from build123d import *

# Parameters (mm, degrees)
ESBO_O1_R                = 2
RESSALTO_EXTRUS_O1_DEPTH = 3.5
ESBO_O2_R                = 1
CORTE_EXTRUS_O1_DEPTH    = 6.573642863


with BuildPart() as part:
    # Esboço1 → Ressalto-extrusão1 (new body)
    with BuildSketch(Plane.XY):
        Circle(ESBO_O1_R)
        with BuildLine():
            ThreePointArc((-1.509485071, 1.312042233), (-1.175570505, 1.618033989), (-0.781369776, 1.84104896))
            Line((-0.781369776, 1.84104896), (-0.871690079, 1.965364192))
            ThreePointArc((-0.871690079, 1.965364192), (-1.253664041, 2.349535361), (-1.734231738, 2.599627912))
            ThreePointArc((-1.734231738, 2.599627912), (-1.836828913, 2.528178107), (-1.936485986, 2.452681599))
            ThreePointArc((-1.936485986, 2.452681599), (-1.847137421, 1.918351711), (-1.599805374, 1.436357465))
            Line((-1.599805374, 1.436357465), (-1.509485071, 1.312042233))
        make_face()
        with BuildLine():
            ThreePointArc((-0.45, 1.948717527), (0, 2), (0.45, 1.948717527))
            Line((0.45, 1.948717527), (0.45, 2.102379604))
            ThreePointArc((0.45, 2.102379604), (0.36678672, 2.63769927), (0.125, 3.122498999))
            ThreePointArc((0.125, 3.122498999), (0, 3.125), (-0.125, 3.122498999))
            ThreePointArc((-0.125, 3.122498999), (-0.36678672, 2.63769927), (-0.45, 2.102379604))
            Line((-0.45, 2.102379604), (-0.45, 1.948717527))
        make_face()
        with BuildLine():
            Line((0.871690079, 1.965364192), (0.781369776, 1.84104896))
            ThreePointArc((0.781369776, 1.84104896), (1.175570505, 1.618033989), (1.509485071, 1.312042233))
            Line((1.509485071, 1.312042233), (1.599805374, 1.436357465))
            ThreePointArc((1.599805374, 1.436357465), (1.847137421, 1.918351711), (1.936485986, 2.452681599))
            ThreePointArc((1.936485986, 2.452681599), (1.836828913, 2.528178107), (1.734231738, 2.599627912))
            ThreePointArc((1.734231738, 2.599627912), (1.253664041, 2.349535361), (0.871690079, 1.965364192))
        make_face()
        with BuildLine():
            Line((1.860424175, 1.077646459), (1.714282855, 1.030162265))
            ThreePointArc((1.714282855, 1.030162265), (1.902113033, 0.618033989), (1.99239815, 0.174211401))
            Line((1.99239815, 0.174211401), (2.13853947, 0.221695594))
            ThreePointArc((2.13853947, 0.221695594), (2.621944409, 0.466259001), (3.008300145, 0.846023191))
            ThreePointArc((3.008300145, 0.846023191), (2.972051613, 0.965678107), (2.931045896, 1.08378732))
            ThreePointArc((2.931045896, 1.08378732), (2.395257749, 1.163928801), (1.860424175, 1.077646459))
        make_face()
        with BuildLine():
            Line((2.13853947, -0.221695594), (1.99239815, -0.174211401))
            ThreePointArc((1.99239815, -0.174211401), (1.902113033, -0.618033989), (1.714282855, -1.030162265))
            Line((1.714282855, -1.030162265), (1.860424175, -1.077646459))
            ThreePointArc((1.860424175, -1.077646459), (2.395257749, -1.163928801), (2.931045896, -1.08378732))
            ThreePointArc((2.931045896, -1.08378732), (2.972051613, -0.965678107), (3.008300145, -0.846023191))
            ThreePointArc((3.008300145, -0.846023191), (2.621944409, -0.466259001), (2.13853947, -0.221695594))
        make_face()
        with BuildLine():
            Line((1.599805374, -1.436357465), (1.509485071, -1.312042233))
            ThreePointArc((1.509485071, -1.312042233), (1.175570505, -1.618033989), (0.781369776, -1.84104896))
            Line((0.781369776, -1.84104896), (0.871690079, -1.965364192))
            ThreePointArc((0.871690079, -1.965364192), (1.253664041, -2.349535361), (1.734231738, -2.599627912))
            ThreePointArc((1.734231738, -2.599627912), (1.836828913, -2.528178107), (1.936485986, -2.452681599))
            ThreePointArc((1.936485986, -2.452681599), (1.847137421, -1.918351711), (1.599805374, -1.436357465))
        make_face()
        with BuildLine():
            Line((0.45, -2.102379604), (0.45, -1.948717527))
            ThreePointArc((0.45, -1.948717527), (0, -2), (-0.45, -1.948717527))
            Line((-0.45, -1.948717527), (-0.45, -2.102379604))
            ThreePointArc((-0.45, -2.102379604), (-0.36678672, -2.63769927), (-0.125, -3.122498999))
            ThreePointArc((-0.125, -3.122498999), (0, -3.125), (0.125, -3.122498999))
            ThreePointArc((0.125, -3.122498999), (0.36678672, -2.63769927), (0.45, -2.102379604))
        make_face()
        with BuildLine():
            ThreePointArc((-0.781369776, -1.84104896), (-1.175570505, -1.618033989), (-1.509485071, -1.312042233))
            Line((-1.509485071, -1.312042233), (-1.599805374, -1.436357465))
            ThreePointArc((-1.599805374, -1.436357465), (-1.847137421, -1.918351711), (-1.936485986, -2.452681599))
            ThreePointArc((-1.936485986, -2.452681599), (-1.836828913, -2.528178107), (-1.734231738, -2.599627912))
            ThreePointArc((-1.734231738, -2.599627912), (-1.253664041, -2.349535361), (-0.871690079, -1.965364192))
            Line((-0.871690079, -1.965364192), (-0.781369776, -1.84104896))
        make_face()
        with BuildLine():
            ThreePointArc((-1.714282855, -1.030162265), (-1.902113033, -0.618033989), (-1.99239815, -0.174211401))
            Line((-1.99239815, -0.174211401), (-2.13853947, -0.221695594))
            ThreePointArc((-2.13853947, -0.221695594), (-2.621944409, -0.466259001), (-3.008300145, -0.846023191))
            ThreePointArc((-3.008300145, -0.846023191), (-2.972051613, -0.965678107), (-2.931045896, -1.08378732))
            ThreePointArc((-2.931045896, -1.08378732), (-2.395257749, -1.163928801), (-1.860424175, -1.077646459))
            Line((-1.860424175, -1.077646459), (-1.714282855, -1.030162265))
        make_face()
        with BuildLine():
            ThreePointArc((-1.99239815, 0.174211401), (-1.902113033, 0.618033989), (-1.714282855, 1.030162265))
            Line((-1.714282855, 1.030162265), (-1.860424175, 1.077646459))
            ThreePointArc((-1.860424175, 1.077646459), (-2.395257749, 1.163928801), (-2.931045896, 1.08378732))
            ThreePointArc((-2.931045896, 1.08378732), (-2.972051613, 0.965678107), (-3.008300145, 0.846023191))
            ThreePointArc((-3.008300145, 0.846023191), (-2.621944409, 0.466259001), (-2.13853947, 0.221695594))
            Line((-2.13853947, 0.221695594), (-1.99239815, 0.174211401))
        make_face()
    extrude(amount=RESSALTO_EXTRUS_O1_DEPTH)

    # Esboço2 → Corte-extrusão1 (cut, through all)
    with BuildSketch(Plane.XY.offset(3.5)):
        Circle(ESBO_O2_R)
    extrude(amount=-CORTE_EXTRUS_O1_DEPTH, mode=Mode.SUBTRACT)


solid = part.part
Can you work these out from the model? Positions are in its coordinate system, mm. A direction names the side the tool comes from. Give positions to 0.01 mm unless a question says otherwise; leave off trailing zeros. Write each loop counter-clockwise with the first axis right and the second up, starting at its lowest first coordinate (ties: lowest second). Pieces come first, ordered by that corner, then holes. Notation, with made-up numbers: M 31,50 L 72,50 A34 ccw 72,87 Z; hole C 4.25,3 d5. An arc over 180 degrees is marked long. Answer in a Markdown table with one row per item. Add a question column.
Item 1: Imagine slicing it at D-D, the plane y = -1.75. Write out the boundary of the cut face in (x, z).
Item 2: We'd pull the mould along X, two halves only. Please class faces 1 (the cylindrical face through (-0.37, -2.63, 1.73)), 2 (the flat face through (-1, 1, 3.5)), 3 (the cylindrical face through (2.63, -0.47, 1.73)), 4 (the cylindrical face through (-1.248, 2.345, 1.726)): released by +X, released by -X, zero draft, split by the parting line, or undercut.
Item 3: On a 3-axis mill with a long thin cutter (end or side, diameter ignored), from which of +Z, -Z, +X, -X, +Y, -Y can I reach the whole of each face in a straight line? I mean faces 5 (the cylindrical face through (-1.845, -1.911, 1.726)), 6 (the cylindrical face through (2.616, 0.462, 1.726)), 7 (the cylindrical face through (1.26, 2.354, 1.726)). Say none if no direction works.
Item 4: Imagine slicing it at B-B, the plane y = 2.25. Write out the boundary of the cut face in (x, z).
Item 5: For pin 1 Ø1.5 at (x, z) = (1, 0.5) entering from -Y, with a flat end and sliding along its axis, tell me the tip position at first contact or that it passes through.
Item 6: Please list where these lines run through material, in increasing order: L1, parallel to X at y = 2, z = 2.45; L2, parallel to Y at x = 0, z = 1.35 (3 decimals).
Item 7: Imagine slicing it at C-C, the plane y = -0.5. Write out the boundary of the cut face in (x, z), plus the area to 3 significant figures.
Item 8: Imagine slicing it at A-A, the plane x = 0. Write out the boundary of the cut face in (y, z) (3 decimals), plus the area to 3 significant figures.
Evaluation:
| question | item | result |
|---|---|---|
| 1 | outline | M -1.78,0 L 1.78,0 L 1.78,3.5 L -1.78,3.5 Z |
| 2 | face 1 | undercut |
| 2 | face 2 | zero draft |
| 2 | face 3 | released by +X |
| 2 | face 4 | undercut |
| 3 | face 5 | +Z, -Z, -X |
| 3 | face 6 | +Z, -Z, +X |
| 3 | face 7 | +Z, -Z, +Y |
| 4 | outline | M -1.92,0 L -1.13,0 L -1.13,3.5 L -1.92,3.5 Z; M -0.44,0 L 0.44,0 L 0.44,3.5 L -0.44,3.5 Z; M 1.13,0 L 1.92,0 L 1.92,3.5 L 1.13,3.5 Z |
| 5 | pin 1 | stops at y = -2.92 |
| 6 | L1 | x = -1.87 to -0.9, -0.45 to 0.45, 0.9 to 1.87 |
| 6 | L2 | y = -3.125 to -1, 1 to 3.125 |
| 7 | outline | M -2.67,0 L -0.87,0 L -0.87,3.5 L -2.67,3.5 Z; M 0.87,0 L 2.67,0 L 2.67,3.5 L 0.87,3.5 Z |
| 7 | area | 12.6 mm² |
| 8 | outline | M -3.125,0 L -1,0 L -1,3.5 L -3.125,3.5 Z; M 1,0 L 3.125,0 L 3.125,3.5 L 1,3.5 Z |
| 8 | area | 14.9 mm² |
